```python
from build123d import *

# Parameters (mm, degrees)
BOX_W             = 4
BOX_H             = 3
BOX_DEPTH         = 2
BOX_ROLL_ANGLE    = -45
CYLINDER001_R     = 0.3
CYLINDER001_DEPTH = 11
CYLINDER_R        = 2
CYLINDER_DEPTH    = 8
CYLINDER002_R     = 0.5
CYLINDER002_DEPTH = 2
PAD_DEPTH         = 2


with BuildPart() as obj1:
    # Box → Box (new body)
    with BuildSketch(Plane.XY):
        with Locations((2, 1.5)):
            Rectangle(BOX_W, BOX_H)
    extrude(amount=BOX_DEPTH)


with BuildPart() as obj1_1:
    # Box roll: moved
    add(obj1.part.rotate(Axis((0, 0, 0), (1, 0, 0)), BOX_ROLL_ANGLE))


with BuildPart() as obj1_2:
    # Box placement: moved
    add(obj1_1.part.moved(Location((-1, 0, 11))))


with BuildPart() as achse:
    # Cylinder001 → Cylinder001 (new body)
    with BuildSketch(Plane.XY):
        Circle(CYLINDER001_R)
    extrude(amount=CYLINDER001_DEPTH)


with BuildPart() as motor:
    # Cylinder → Cylinder (new body)
    with BuildSketch(Plane.XY):
        Circle(CYLINDER_R)
    extrude(amount=CYLINDER_DEPTH)


with BuildPart() as zylinder:
    # Cylinder002 → Cylinder002 (new body)
    with BuildSketch(Plane.XY.offset(9)):
        Circle(CYLINDER002_R)
    extrude(amount=CYLINDER002_DEPTH)


with BuildPart() as cut:
    # Sketch → Pad (new body)
    with BuildSketch(Plane.XY.offset(9)):
        with BuildLine():
            Line((0, 2), (0, -2))
            ThreePointArc((0, -2), (2, 0), (0, 2))
        make_face()
    extrude(amount=PAD_DEPTH)

    # Fusion: union Achse, Motor, Zylinder
    add(achse.part)
    add(motor.part)
    add(zylinder.part)

    # Cut: cut obj1
    add(obj1_2.part, mode=Mode.SUBTRACT)


solid = cut.part
```
CAD build for the part. Positions are in the model's coordinates, mm. A direction names the side the tool comes from. Round coordinates to 2 decimals unless told otherwise and drop trailing zeros. Loops run counter-clockwise (first coordinate to the right, second up) from the corner with the lowest first, then second, coordinate; pieces in that order, holes last. Notation, with made-up numbers: M 16,-14 L 24,-14 A7 ccw 24,-1 Z; hole C 83,51.5 d5. An arc over 180 degrees is marked long. Return JSON: item names as keys, results as strings. Group by question number.
(1) Saw through at B-B, the plane x = 0.85. List the corners of the cut face in (y, z), and give its area (3 significant figures).
(2) Mould opens along Z. For faces 4 (the flat face through (0, 0.5, 8)), 5 (the cylindrical face through (0, -2, 4)), 6 (the flat face through (1, 1, 10)), 7 (the flat face through (1, 0, 9)) say: +Z half, -Z half, draft (parallel to the pull), parting line (faces both ways), or undercut.
(3) Tool access for faces 1 (the flat face through (0, 0.9, 9.4)), 2 (the flat face through (0, -1, 10)), 3 (the cylindrical face through (-0.5, 0, 10)): list every direction of +Z, -Z, +X, -X, +Y, -Y with a clear straight run to the whole face (end or side of a thin tool).
(4) Saw through at A-A, the plane y = 1.45. List the corners of the cut face in (x, z), and give its area (3 significant figures).
(5) Drop flat-ended pins along their axis: P1, Ø1.6, axis at y = 1, z = 10, coming from the -X side; P2, Ø2, axis at x = -1.5, y = 1, coming from the +Z side; P3, Ø1.2, axis at x = 1, y = -0.5, coming from the -Z side; P4, Ø1.5, axis at x = 1.5, z = 8.5, coming from the -Y side. Give the stop position or say it passes through.
(6) Saw through at D-D, the plane z = 10. List the corners of the cut face in (x, y).
(7) Wall check: probe 1 along Z at (x, y) = (0.35, -1.4); probe 2 along Z at (x, y) = (0.85, 0.5); probe 3 along X at (y, z) = (0, 8.75). Give the ranges that are in metal, low to high. Write a range as [from, to].
Answer list:
{
 "1": {"outline": "M -1.81,0 L 1.81,0 L 1.81,8 L -1.81,8 Z; M -1.81,9 L 1.81,9 L 1.81,9.19 L 0,11 L -1.81,11 Z", "area": "34.6 mm2"},
 "2": {"face 4": "undercut", "face 5": "draft", "face 6": "+Z half", "face 7": "undercut"},
 "3": {"face 1": "+Z, -X, +Y", "face 2": "+Z, -X, -Y", "face 3": "+Z, -X"},
 "4": {"outline": "M -1.38,0 L 1.38,0 L 1.38,8 L -1.38,8 Z; M 0,9 L 1.38,9 L 1.38,9.55 L 0,9.55 Z", "area": "22.8 mm2"},
 "5": {"P1": "x = -0.46", "P2": "z = 8", "P3": "z = 0", "P4": "y = -1.76"},
 "6": {"outline": "M 0,-2 A2 ccw 1.73,1 L 0,1 L 0,0.5 A0.5 ccw 0,-0.5 Z"},
 "7": {"probe 1": "[0, 8], [9, 11]", "probe 2": "[0, 8], [9, 10.5]", "probe 3": "[-0.3, 0.3]"}
}
